from build123d import *

# Parameters (mm, degrees)
F0_W      = 31.75
F0_H      = 25.4
F1_DEPTH  = 25.4
F2_W      = 6.35
F2_H      = 12.7
F3_DEPTH  = 25.4
F4_DEPTH  = 25.4
F5_W      = 19.05
F5_H      = 12.7
F6_DEPTH  = 25.4
F7_R      = 6.35
F8_DEPTH  = 12.7
F10_DEPTH = 25.4


with BuildPart() as f1:
    # F0 (on Front) → F1 (new body)
    with BuildSketch(Plane.XZ):
        with Locations((15.875, 12.7)):
            Rectangle(F0_W, F0_H)
    extrude(amount=F1_DEPTH)

    # F2 (on face) → F3 (cut)
    with BuildSketch(Plane.YZ.offset(31.75)):
        with Locations((-22.225, 12.7)):
            Rectangle(F2_W, F2_H)
    extrude(amount=-F3_DEPTH, mode=Mode.SUBTRACT)

    # F4 (cut): a face of the model
    f4_faces = [f1.faces().sort_by_distance(p)[0] for p in [
        (6.35, -22.225, 12.7),
    ]]
    extrude(f4_faces, amount=-F4_DEPTH, mode=Mode.SUBTRACT)

    # F5 (on face) → F6 (cut)
    with BuildSketch(Plane.XY.offset(25.4)):
        with Locations((22.225, -19.05)):
            Rectangle(F5_W, F5_H)
    extrude(amount=-F6_DEPTH, mode=Mode.SUBTRACT)

    # F7 (on face) → F8 (cut, through all)
    with BuildSketch(Plane.XZ.offset(12.7)):
        with Locations((20.9659710526, 12.7)):
            Circle(F7_R)
    extrude(amount=-F8_DEPTH, mode=Mode.SUBTRACT)

    # F9 (on face) → F10 (cut)
    with BuildSketch(Plane.XZ.offset(12.7)):
        with BuildLine():
            ThreePointArc((22.225, 25.4), (31.3787710318, 12.7), (22.225, 0))
            Line((22.225, 0), (31.75, 0))
            Line((31.75, 0), (31.75, 25.4))
            Line((31.75, 25.4), (22.225, 25.4))
        make_face()
    extrude(amount=-F10_DEPTH, mode=Mode.SUBTRACT)


solid = f1.part
Work out the finished part from the listing and answer in its coordinate system (mm). A direction names the side the tool comes from. Give positions to 0.01 mm unless a question says otherwise; leave off trailing zeros. Loops run counter-clockwise (first coordinate to the right, second up) from the corner with the lowest first, then second, coordinate; pieces in that order, holes last. Notation, with made-up numbers: (8.5, 28) - (33.5, 28) arc R15 ccw to (33.5, 46) - close; hole circle Ø9 at (-8.75, 88). An arc over 180 degrees is marked (long way). Answer in a Markdown table with one row per item.
(1) Section D-D (x = 12) is taken. Give the vertices of the cut face in (y, z), and give its area (3 significant figures).
Results list:
| item | result |
|---|---|
| outline | (-25.4, 0) - (0, 0) - (0, 25.4) - (-25.4, 25.4) - (-25.4, 19.05) - (-19.05, 19.05) - (-19.05, 6.35) - (-25.4, 6.35) - close |
| area | 565 mm² |
(2) Section A-A (z = 12.7) is taken. Give the vertices of the cut face in (x, y).
Results list:
| item | result |
|---|---|
| outline | (0, -19.05) - (12.7, -19.05) - (12.7, -12.7) - (14.62, -12.7) - (14.62, 0) - (0, 0) - close; (27.32, -12.7) - (31.38, -12.7) - (31.38, 0) - (27.32, 0) - close |
(3) Flat-ended cylindrical pins translate along their axes: pin 1 Ø3 at (x, z) = (23, 22.5) entering from -Y; pin 2 Ø4 at (x, y) = (24, -14) entering from +Z; pin 3 Ø2 at (x, z) = (10, 8.5) entering from -Y. Find the tip coordinate at first contact, or state that the pin passes through.
Results list:
| item | result |
|---|---|
| pin 1 | stops at y = -12.7 |
| pin 2 | stops at z = 25.31 |
| pin 3 | stops at y = -19.05 |
(4) Consider L1, parallel to Z at x = 5, y = -24; L2, parallel to Y at x = 15.5, z = 19.5; L3, parallel to Y at x = 2.5, z = 14.5. Determine where each line is inside the solid, lowest interval first. Write a range as [from, to].
Results list:
| item | result |
|---|---|
| L1 | z = [0, 6.35], [19.05, 25.4] |
| L2 | y = [-12.7, 0] |
| L3 | y = [-19.05, 0] |
(5) Section B-B (x = 18) is taken. Give the vertices of the cut face in (y, z).
Results list:
| item | result |
|---|---|
| outline | (-12.7, 0) - (0, 0) - (0, 7.09) - (-12.7, 7.09) - close; (-12.7, 18.31) - (0, 18.31) - (0, 25.4) - (-12.7, 25.4) - close |
(6) A tool of negligible diameter and unlimited length cuts with its end or side. For faces 1 (the face through (6, -22, 19.05)), 2 (the face through (16.286, -6.439, 16.992)), 3 (the face through (24, -12.7, 19)), from which of +Z, -Z, +X, -X, +Y, -Y can it reach the whole face along a straight path? Write none if from no direction.
Results list:
| item | result |
|---|---|
| face 1 | +X, -X, -Y |
| face 2 | +Y, -Y |
| face 3 | +Z, -Z, +X, -Y |
(7) Section C-C (y = -12) is taken. Give the vertices of the cut face in (x, z) (3 decimals).
Results list:
| item | result |
|---|---|
| outline | (0, 0) - (22.225, 0) arc R13.387 ccw to (22.225, 25.4) - (0, 25.4) - close; hole circle Ø12.7 at (20.966, 12.7) |
(8) For a pull along Z with two mould halves and no side action, classify faces 4 (the face through (6, -22, 6.35)), 5 (the face through (31.377, -6.439, 12.934)), 6 (the face through (12, 0, 13)) as pulls with the +Z half, pulls with the -Z half, needs draft (parallel to the pull), parting line crosses it, or undercut.
Results list:
| item | result |
|---|---|
| face 4 | undercut |
| face 5 | parting line crosses it |
| face 6 | needs draft |
